```python
from build123d import *

# Parameters (mm, degrees)
BOX002_W     = 50
BOX002_H     = 3
BOX002_DEPTH = 1
BOX001_W     = 50
BOX001_H     = 4
BOX001_DEPTH = 1
BOX_W        = 50
BOX_H        = 14.5
BOX_DEPTH    = 10
BOX003_W     = 10
BOX003_H     = 5
BOX003_DEPTH = 16


with BuildPart() as cube002:
    # Box002 → Box002 (new body)
    with BuildSketch(Plane(origin=(0, 11.5, 4.5), x_dir=(1, 0, 0), z_dir=(0, 0, 1))):
        with Locations((25, 1.5)):
            Rectangle(BOX002_W, BOX002_H)
    extrude(amount=BOX002_DEPTH)


with BuildPart() as cube001:
    # Box001 → Box001 (new body)
    with BuildSketch(Plane.XY.offset(4.5)):
        with Locations((25, 2)):
            Rectangle(BOX001_W, BOX001_H)
    extrude(amount=BOX001_DEPTH)


with BuildPart() as cut001:
    # Box → Box (new body)
    with BuildSketch(Plane.XY):
        with Locations((25, 7.25)):
            Rectangle(BOX_W, BOX_H)
    extrude(amount=BOX_DEPTH)

    # Cut: cut Cube001
    add(cube001.part, mode=Mode.SUBTRACT)

    # Cut001: cut Cube002
    add(cube002.part, mode=Mode.SUBTRACT)


with BuildPart() as test_slider001:
    # Box003 → Box003 (new body)
    with BuildSketch(Plane(origin=(0, 5, 0), x_dir=(1, 0, 0), z_dir=(0, 0, 1))):
        with Locations((5, 2.5)):
            Rectangle(BOX003_W, BOX003_H)
    extrude(amount=BOX003_DEPTH)

    # Fusion: union Cut001
    add(cut001.part)


solid = test_slider001.part
```
Work out the finished part from the listing and answer in its coordinate system (mm). A direction names the side the tool comes from. Round coordinates to 2 decimals unless told otherwise and drop trailing zeros. Loops run counter-clockwise (first coordinate to the right, second up) from the corner with the lowest first, then second, coordinate; pieces in that order, holes last. Notation, with made-up numbers: (64.25, 49) -> (89.25, 49) arc R12 cw to (89.25, 54) -> close; hole circle Ø2 at (-16, -3). An arc over 180 degrees is marked (long way). Write each question's results on one line, items separated by ' | '. Start each with the question number.
1. Section B-B (x = 9.5) is taken. Determine the outline of the cut face in (y, z).
2. For a pull along Z with two mould halves and no side action, classify faces 1 (the face through (5, 8, 16)), 2 (the face through (25, 11.5, 5)), 3 (the face through (50, 7, 5)) as +Z half, -Z half, draft (parallel to the pull), parting line (faces both ways), or undercut.
3. A tool of negligible diameter and unlimited length cuts with its end or side. For faces 4 (the face through (25, 2, 5.5)), 5 (the face through (10, 7, 13)), 6 (the face through (25, 13, 5.5)), 7 (the face through (5, 5, 13)), from which of +Z, -Z, +X, -X, +Y, -Y can it reach the whole face along a straight path? Write none if from no direction.
4. Section C-C (z = 14) is taken. Determine the outline of the cut face in (x, y).
5. Given pin 1 Ø5 at (x, z) = (7.5, 14.5) entering from +Y; pin 2 Ø5.5 at (y, z) = (8.5, 14.5) entering from +X; pin 3 Ø0.5 at (x, z) = (16, 5) entering from -Y, each flat-ended and moving along its own axis, determine where each tip first touches the part or whether it passes through.
6. Section A-A (y = 12.5) is taken. Determine the outline of the cut face in (x, z).
7. Find the intervals of material crossed by probe 1 along Z at (x, y) = (19.5, 1.75); probe 2 along X at (y, z) = (6.75, 10.5), in increasing order. Write a range as from..to.
8. Section D-D (y = 7.25) is taken. Determine the outline of the cut face in (x, z).
Evaluation:
1) outline: (0, 0) -> (14.5, 0) -> (14.5, 4.5) -> (11.5, 4.5) -> (11.5, 5.5) -> (14.5, 5.5) -> (14.5, 10) -> (10, 10) -> (10, 16) -> (5, 16) -> (5, 10) -> (0, 10) -> (0, 5.5) -> (4, 5.5) -> (4, 4.5) -> (0, 4.5) -> close
2) face 1: +Z half | face 2: undercut | face 3: draft
3) face 4: +X, -X, -Y | face 5: +Z, +X, +Y, -Y | face 6: +X, -X, +Y | face 7: +Z, +X, -X, -Y
4) outline: (0, 5) -> (10, 5) -> (10, 10) -> (0, 10) -> close
5) pin 1: stops at y = 10 | pin 2: stops at x = 10 | pin 3: stops at y = 4
6) outline: (0, 0) -> (50, 0) -> (50, 4.5) -> (0, 4.5) -> close; (0, 5.5) -> (50, 5.5) -> (50, 10) -> (0, 10) -> close
7) probe 1: z = 0..4.5, 5.5..10 | probe 2: x = 0..10
8) outline: (0, 0) -> (50, 0) -> (50, 10) -> (10, 10) -> (10, 16) -> (0, 16) -> close
